Can you work these out from the model? Positions are in its coordinate system, mm. A direction names the side the tool comes from. Round coordinates to 2 decimals unless told otherwise and drop trailing zeros. Write each loop counter-clockwise with the first axis right and the second up, starting at its lowest first coordinate (ties: lowest second). Pieces come first, ordered by that corner, then holes.
Q1. If we section it at B-B (x = -10): Please give me the cut outline in (y, z).
Q2. If we section it at D-D (x = -15): Please give me the cut outline in (y, z).
Q3. If we section it at C-C (y = -5): Please give me the cut outline in (x, z).
Q4. I'm going to push flat-ended pins straight in: pin 1 Ø1.6 at (y, z) = (-5.5, 4) entering from -X; pin 2 Ø1.6 at (y, z) = (-4.5, 6) entering from +X; pin 3 Ø3 at (x, z) = (-5, 5) entering from -Y. Where does each tip first touch, or does it pass through?
Q5. If we section it at A-A (z = 14): Please give me the cut outline in (x, y), plus the area to 3 significant figures.
Q6. We'd pull the mould along X, two halves only. Please class faces 1 (the cylindrical face through (-19.51, -9.44, 7.46)), 2 (the flat face through (-19, -10, 10)), 3 (the flat face through (-10, -19, 10)), 4 (the flat face through (-1, -15, 5)): +X half, -X half, draft (parallel to the pull), parting line (faces both ways), or undercut.
Q7. For faces 5 (the flat face through (-1, -5, 15)), 6 (the cylindrical face through (-3.8, -19.507, 12.693)), 7 (the flat face through (-15, -1, 15)), which set-ups out of +Z, -Z, +X, -X, +Y, -Y let a thin tool reach every point of the face, with its end or its side?
Q8. Please list where these lines run through material, in increasing order: line 1 along Z through (x, y) = (-0.55, -15); line 2 along Z through (x, y) = (-5, -0.8); line 3 along Y through (x, z) = (-0.75, 13.25).
from build123d import *

# Parameters (mm, degrees)
F0_W      = 20
F0_H      = 20
F1_DEPTH  = 20
F2_R      = 2.6
F3_DEPTH  = 1
F4_R      = 2.6
F5_DEPTH  = 1
F6_R      = 2.6
F7_DEPTH  = 1
F8_R      = 2.6
F9_DEPTH  = 1
F10_R     = 2.6
F11_DEPTH = 1


with BuildPart() as f1:
    # F0 (on Front) → F1 (new body)
    with BuildSketch(Plane.XZ):
        with Locations((-10, 10)):
            Rectangle(F0_W, F0_H)
    extrude(amount=F1_DEPTH)

    # F2 (on face) → F3 (cut)
    with BuildSketch(Plane.XZ.offset(20)):
        with Locations((-15, 15)):
            Circle(F2_R)
        with Locations((-10, 10)):
            Circle(F2_R)
        with Locations((-15, 5)):
            Circle(F2_R)
        with Locations((-5, 15)):
            Circle(F2_R)
        with Locations((-5, 5)):
            Circle(F2_R)
    extrude(amount=-F3_DEPTH, mode=Mode.SUBTRACT)

    # F4 (on face) → F5 (cut)
    with BuildSketch(Plane(origin=(0, 0, 0), x_dir=(-1, 0, 0), z_dir=(0, 1, 0))):
        with Locations((15, 15)):
            Circle(F4_R)
        with Locations((5, 5)):
            Circle(F4_R)
    extrude(amount=-F5_DEPTH, mode=Mode.SUBTRACT)

    # F6 (on face) → F7 (cut)
    with BuildSketch(Plane.XY.offset(20)):
        with Locations((-10, -10)):
            Circle(F6_R)
    extrude(amount=-F7_DEPTH, mode=Mode.SUBTRACT)

    # F8 (on face) → F9 (cut)
    with BuildSketch(Plane(origin=(-20, 0, 0), x_dir=(0, -1, 0), z_dir=(-1, 0, 0))):
        with Locations((10, 10)):
            Circle(F8_R)
        with Locations((15, 15)):
            Circle(F8_R)
        with Locations((5, 5)):
            Circle(F8_R)
    extrude(amount=-F9_DEPTH, mode=Mode.SUBTRACT)

    # F10 (on face) → F11 (cut)
    with BuildSketch(Plane.YZ):
        with Locations((-15, 15)):
            Circle(F10_R)
        with Locations((-15, 5)):
            Circle(F10_R)
        with Locations((-5, 15)):
            Circle(F10_R)
        with Locations((-5, 5)):
            Circle(F10_R)
    extrude(amount=-F11_DEPTH, mode=Mode.SUBTRACT)


solid = f1.part
A:
1. outline: (-20, 0) - (0, 0) - (0, 20) - (-7.4, 20) - (-7.4, 19) - (-12.6, 19) - (-12.6, 20) - (-20, 20) - (-20, 12.6) - (-19, 12.6) - (-19, 7.4) - (-20, 7.4) - close
2. outline: (-20, 0) - (0, 0) - (0, 12.4) - (-1, 12.4) - (-1, 17.6) - (0, 17.6) - (0, 20) - (-20, 20) - (-20, 17.6) - (-19, 17.6) - (-19, 12.4) - (-20, 12.4) - (-20, 7.6) - (-19, 7.6) - (-19, 2.4) - (-20, 2.4) - close
3. outline: (-20, 0) - (0, 0) - (0, 2.4) - (-1, 2.4) - (-1, 7.6) - (0, 7.6) - (0, 12.4) - (-1, 12.4) - (-1, 17.6) - (0, 17.6) - (0, 20) - (-20, 20) - (-20, 7.6) - (-19, 7.6) - (-19, 2.4) - (-20, 2.4) - close
4. pin 1: stops at x = -19
4. pin 2: stops at x = -1
4. pin 3: stops at y = -19
5. outline: (-20, -20) - (-17.4, -20) - (-17.4, -19) - (-12.6, -19) - (-12.6, -20) - (-7.4, -20) - (-7.4, -19) - (-2.6, -19) - (-2.6, -20) - (0, -20) - (0, -17.4) - (-1, -17.4) - (-1, -12.6) - (0, -12.6) - (0, -7.4) - (-1, -7.4) - (-1, -2.6) - (0, -2.6) - (0, 0) - (-12.6, 0) - (-12.6, -1) - (-17.4, -1) - (-17.4, 0) - (-20, 0) - (-20, -12.6) - (-19, -12.6) - (-19, -17.4) - (-20, -17.4) - close
5. area: 371 mm2
6. face 1: draft
6. face 2: -X half
6. face 3: undercut
6. face 4: +X half
7. face 5: +X
7. face 6: -Y
7. face 7: +Y
8. line 1: z = 0 to 2.4, 7.6 to 12.4, 17.6 to 20
8. line 2: z = 0 to 2.4, 7.6 to 20
8. line 3: y = -20 to -16.92, -13.08 to -6.92, -3.08 to 0
